```python
from build123d import *

# Parameters (mm, degrees)
F0_W     = 90
F0_H     = 59.5
F1_DEPTH = 3
F2_W     = 11
F2_H     = 24
F3_DEPTH = 41
F2_W_2   = 6
F2_H_2   = 56
F4_DEPTH = 31
F5_W     = 18
F5_H     = 11
F6_DEPTH = 15
F8_DEPTH = 10


with BuildPart() as f1:
    # F0 (on Top) → F1 (new body)
    with BuildSketch(Plane.XY):
        with Locations((45, 29.3979640784)):
            Rectangle(F0_W, F0_H)
    extrude(amount=F1_DEPTH)

    # F2 (on face) → F3 (join)
    with BuildSketch(Plane.XY.offset(3)):
        with Locations((26.5, 29.1479640784)):
            Rectangle(F2_W, F2_H)
    extrude(amount=F3_DEPTH)

    # F2 (on face) → F4 (join)
    with BuildSketch(Plane.XY.offset(3)):
        with Locations((62, 29.6479640784)):
            Rectangle(F2_W_2, F2_H_2)
    extrude(amount=F4_DEPTH)

    # F5 (on face) → F6 (cut)
    with BuildSketch(Plane(origin=(21, 0, 0), x_dir=(0, -1, 0), z_dir=(-1, 0, 0))):
        Polygon((-41.1479640784, 27), (-41.1479640784, 3), (-38.1479640784, 3), (-38.1479640784, 17), align=None)
        with Locations((-29.1479640784, 35.5)):
            Rectangle(F5_W, F5_H)
        Polygon((-20.1479640784, 17), (-20.1479640784, 3), (-17.1479640784, 3), (-17.1479640784, 27), align=None)
    extrude(amount=-F6_DEPTH, mode=Mode.SUBTRACT)

    # F7 (on face) → F8 (cut)
    with BuildSketch(Plane.YZ.offset(65)):
        with BuildLine():
            Line((29.6479640784, 34), (4.6479640784, 34))
            ThreePointArc((4.6479640784, 34), (7.8351090818, 21.7852811372), (16.5839126302, 12.6849686897))
            Line((16.5839126302, 12.6849686897), (29.6479640784, 34))
        make_face()
        with BuildLine():
            ThreePointArc((16.5839126302, 12.6849686897), (29.6479640784, 9), (42.7120155267, 12.6849686897))
            Line((42.7120155267, 12.6849686897), (29.6479640784, 34))
            Line((29.6479640784, 34), (16.5839126302, 12.6849686897))
        make_face()
        with BuildLine():
            ThreePointArc((42.7120155267, 12.6849686897), (51.460819075, 21.7852811372), (54.6479640784, 34))
            Line((54.6479640784, 34), (29.6479640784, 34))
            Line((29.6479640784, 34), (42.7120155267, 12.6849686897))
        make_face()
        with BuildLine():
            ThreePointArc((16.5839126302, 12.6849686897), (7.8351090818, 21.7852811372), (4.6479640784, 34))
            Line((4.6479640784, 34), (1.6479640784, 34))
            ThreePointArc((1.6479640784, 34), (5.2175664822, 20.3195148737), (15.0162264564, 10.1271649325))
            Line((15.0162264564, 10.1271649325), (16.5839126302, 12.6849686897))
        make_face()
        with BuildLine():
            ThreePointArc((15.0162264564, 10.1271649325), (5.2175664822, 20.3195148737), (1.6479640784, 34))
            Line((1.6479640784, 34), (1.6479640784, 3))
            Line((1.6479640784, 3), (10.6479640784, 3))
            Line((10.6479640784, 3), (15.0162264564, 10.1271649325))
        make_face()
        with BuildLine():
            Line((57.6479640784, 3), (57.6479640784, 34))
            ThreePointArc((57.6479640784, 34), (54.0783616746, 20.3195148737), (44.2797017005, 10.1271649325))
            Line((44.2797017005, 10.1271649325), (48.6479640784, 3))
            Line((48.6479640784, 3), (57.6479640784, 3))
        make_face()
        with BuildLine():
            Line((57.6479640784, 34), (54.6479640784, 34))
            ThreePointArc((54.6479640784, 34), (51.460819075, 21.7852811372), (42.7120155267, 12.6849686897))
            Line((42.7120155267, 12.6849686897), (44.2797017005, 10.1271649325))
            ThreePointArc((44.2797017005, 10.1271649325), (54.0783616746, 20.3195148737), (57.6479640784, 34))
        make_face()
    extrude(amount=-F8_DEPTH, mode=Mode.SUBTRACT)


solid = f1.part
```
Could you check a few things on this model? Use its own coordinates, in mm. A direction names the side the tool comes from. Round coordinates to 2 decimals unless told otherwise and drop trailing zeros. Write each loop counter-clockwise with the first axis right and the second up, starting at its lowest first coordinate (ties: lowest second). Pieces come first, ordered by that corner, then holes.
(1) Suppose I cut it at D-D on z = 15.5. Write out the boundary of the cut face in (x, y).
Findings below:
outline: (21, 20.15) - (32, 20.15) - (32, 38.15) - (21, 38.15) - close
(2) If I drill on probe 1 along X at (y, z) = (37, 3.5); probe 2 along Y at (x, z) = (27, 32); probe 3 along X at (y, z) = (39, 26.5), over which ranges is the centre line in solid material (lowest first)?
Findings below:
probe 1: x = 21 to 32, 59 to 65
probe 2: y = 17.15 to 20.15, 38.15 to 41.15
probe 3: x = 21 to 32
(3) Suppose I cut it at C-C on y = 40. Write out the boundary of the cut face in (x, z).
Findings below:
outline: (0, 0) - (90, 0) - (90, 3) - (65, 3) - (65, 11.24) - (59, 11.24) - (59, 3) - (0, 3) - close; (21, 23.17) - (32, 23.17) - (32, 44) - (21, 44) - close
(4) Suppose I cut it at A-A on z = 31. Write out the boundary of the cut face in (x, y).
Findings below:
outline: (21, 17.15) - (32, 17.15) - (32, 20.15) - (21, 20.15) - close; (21, 38.15) - (32, 38.15) - (32, 41.15) - (21, 41.15) - close
(5) Suppose I cut it at B-B on x = 29. Write out the boundary of the cut face in (y, z).
Findings below:
outline: (-0.35, 0) - (59.15, 0) - (59.15, 3) - (38.15, 3) - (38.15, 17) - (41.15, 27) - (41.15, 44) - (17.15, 44) - (17.15, 27) - (20.15, 17) - (20.15, 3) - (-0.35, 3) - close; hole (20.15, 30) - (38.15, 30) - (38.15, 41) - (20.15, 41) - close
(6) Which directions (+Z, -Z, +X, -X, +Y, -Y) give clear straight access to the entire face, cutting with the end or side of a thin tool? Please do faces 1 (the face through (26.423, 39.627, 21.93)), 2 (the face through (26, 38.148, 10)), 3 (the face through (26, 20.148, 35)), 4 (the face through (26, 17.148, 35)).
Findings below:
face 1: +X, -X, +Y
face 2: -X, +Y
face 3: +X, -X
face 4: +Z, +X, -X, -Y
(7) Thinking about a two-plate mould opening in Y: for faces 5 (the face through (62, 29.5, 9)), 6 (the face through (44, 59.148, 1)), 7 (the face through (21, 29, 23)), which applies, +Y half, -Y half, draft (parallel to the pull), parting line (faces both ways), or undercut?
Findings below:
face 5: undercut
face 6: +Y half
face 7: draft
(8) For pin 1 (5.5 mm diameter, centred on x = 26, z = 34.5, fed in from -Y); pin 2 (3.5 mm diameter, centred on x = 24.5, z = 12, fed in from +Y); pin 3 (9 mm diameter, centred on x = 28, z = 11, fed in from -Y), each with a flat end and sliding along its axis, tell me the tip position at first contact or that it passes through.
Findings below:
pin 1: stops at y = 17.15
pin 2: stops at y = 38.15
pin 3: stops at y = 20.15
